```python
from build123d import *

# Parameters (mm, degrees)
ESBO_O1_R                = 3
RESSALTO_EXTRUS_O1_DEPTH = 30


with BuildPart() as part:
    # Esboço1 → Ressalto-extrusão1 (new body)
    with BuildSketch(Plane.XY):
        with BuildLine():
            Line((4.737261314, 4.494822715), (3.666174209, 6.35))
            Line((3.666174209, 6.35), (1.524, 6.35))
            ThreePointArc((1.524, 6.35), (0, 4.826), (-1.524, 6.35))
            Line((-1.524, 6.35), (-3.666174209, 6.35))
            Line((-3.666174209, 6.35), (-4.737261314, 4.494822715))
            ThreePointArc((-4.737261314, 4.494822715), (-4.179438599, 3.937), (-3.975261314, 3.175))
            ThreePointArc((-3.975261314, 3.175), (-4.737261314, 1.855177285), (-6.261261314, 1.855177285))
            Line((-6.261261314, 1.855177285), (-7.332348419, 0))
            Line((-7.332348419, 0), (-6.261261314, -1.855177285))
            ThreePointArc((-6.261261314, -1.855177285), (-4.737261314, -1.855177285), (-3.975261314, -3.175))
            ThreePointArc((-3.975261314, -3.175), (-4.179438599, -3.937), (-4.737261314, -4.494822715))
            Line((-4.737261314, -4.494822715), (-3.666174209, -6.35))
            Line((-3.666174209, -6.35), (-1.524, -6.35))
            ThreePointArc((-1.524, -6.35), (0, -4.826), (1.524, -6.35))
            Line((1.524, -6.35), (3.666174209, -6.35))
            Line((3.666174209, -6.35), (4.737261314, -4.494822715))
            ThreePointArc((4.737261314, -4.494822715), (4.179438599, -2.413), (6.261261314, -1.855177285))
            Line((6.261261314, -1.855177285), (7.332348419, 0))
            Line((7.332348419, 0), (6.261261314, 1.855177285))
            ThreePointArc((6.261261314, 1.855177285), (4.179438599, 2.413), (4.737261314, 4.494822715))
        make_face()
        Circle(ESBO_O1_R, mode=Mode.SUBTRACT)
    extrude(amount=RESSALTO_EXTRUS_O1_DEPTH)


solid = part.part
```
Geometry: final body of the model. Coordinates: model frame, mm. Coordinates: 2 decimals unless noted, no trailing zeros. Order: outer loops, then holes, each group sorted by start corner. A loop starts at its lowest first (then second) coordinate and runs counter-clockwise, first axis right, second up. Notation, with made-up numbers: M -1,74 L 44,74 A21 cw 44,87 Z; hole C 66.25,40.5 d2. An arc over 180 degrees is marked long. Answer in a Markdown table with one row per item. Add a question column.
Q1. Contact query for flat-ended pins moving along their axis: P1, Ø4, axis at y = -4.5, z = 19.5, coming from the +X side; P2, Ø2, axis at y = -1.5, z = 19.5, coming from the -X side; P3, Ø1.5, axis at x = 0.5, z = 4, coming from the +Y side. Output: stop coordinate, or through.
Q2. Section query A-A on x = 0. Return the cut outline in (y, z), and give its area (3 significant figures).
Q3. Mould query, pull axis X, two halves, no side actions, for faces 1 (the flat face through (6.804, 0.915, 14.79)), 2 (the flat face through (-3, 6.35, 15)), 3 (the flat face through (-4.19, 5.44, 14.79)), 4 (the cylindrical face through (4.163, -2.442, 14.79)). Classes: released by +X, released by -X, zero draft, split by the parting line, or undercut.
Q4. Section query D-D on y = 3.75. Return the cut outline in (x, z), and give its area (3 significant figures).
Q5. Line query: L1, parallel to Y at x = 0, z = 14; L2, parallel to X at y = -0.5, z = 2; L3, parallel to X at y = 5.25, z = 6. Output: solid intervals per line, ascending.
Q6. Section query C-C on z = 23. Return the cut outline in (x, y) (3 decimals).
Q7. Section query B-B on y = -5.5. Return the cut outline in (x, z), and give its area (3 significant figures).
Completed:
| question | item | result |
|---|---|---|
| 1 | P1 | stops at x = 4.74 |
| 1 | P2 | stops at x = -7.04 |
| 1 | P3 | stops at y = 5.48 |
| 2 | outline | M -4.83,0 L -3,0 L -3,30 L -4.83,30 Z; M 3,0 L 4.83,0 L 4.83,30 L 3,30 Z |
| 2 | area | 110 mm2 |
| 3 | face 1 | released by +X |
| 3 | face 2 | zero draft |
| 3 | face 3 | released by -X |
| 3 | face 4 | undercut |
| 4 | outline | M -4.09,0 L 4.09,0 L 4.09,30 L -4.09,30 Z |
| 4 | area | 245 mm2 |
| 5 | L1 | y = -4.83 to -3, 3 to 4.83 |
| 5 | L2 | x = -7.04 to -2.96, 2.96 to 7.04 |
| 5 | L3 | x = -4.3 to -1.05, 1.05 to 4.3 |
| 6 | outline | M -7.332,0 L -6.261,-1.855 A1.524 cw -4.737,-4.495 L -3.666,-6.35 L -1.524,-6.35 A1.524 cw 1.524,-6.35 L 3.666,-6.35 L 4.737,-4.495 A1.524 cw 6.261,-1.855 L 7.332,0 L 6.261,1.855 A1.524 cw 4.737,4.495 L 3.666,6.35 L 1.524,6.35 A1.524 cw -1.524,6.35 L -3.666,6.35 L -4.737,4.495 A1.524 cw -6.261,1.855 Z; hole C 0,0 d6 |
| 7 | outline | M -4.16,0 L -1.26,0 L -1.26,30 L -4.16,30 Z; M 1.26,0 L 4.16,0 L 4.16,30 L 1.26,30 Z |
| 7 | area | 174 mm2 |
